from build123d import *

# Parameters (mm, degrees)
F0_W     = 580
F0_H     = 180
F1_DEPTH = 10
F2_W     = 560
F2_H     = 180
F2_W_2   = 540
F2_H_2   = 160
F3_DEPTH = 5


with BuildPart() as f1:
    # F0 (on Top) → F1 (new body)
    with BuildSketch(Plane.XY):
        Rectangle(F0_W, F0_H)
    extrude(amount=F1_DEPTH)

    # F2 (on face) → F3 (cut)
    with BuildSketch(Plane.XY.offset(10)):
        Rectangle(F2_W, F2_H)
        Rectangle(F2_W_2, F2_H_2, mode=Mode.SUBTRACT)
    extrude(amount=-F3_DEPTH, mode=Mode.SUBTRACT)


solid = f1.part
Can you work these out from the model? Positions are in its coordinate system, mm. Give positions to 0.01 mm unless a question says otherwise; leave off trailing zeros. Loops run counter-clockwise (first coordinate to the right, second up) from the corner with the lowest first, then second, coordinate; pieces in that order, holes last. Notation, with made-up numbers: (45.5, 57.25) -> (59.5, 57.25) arc R8 ccw to (59.5, 65.25) -> close; hole circle Ø9 at (15, 54.5). An arc over 180 degrees is marked (long way). Write item = value, one per line.
1) I need wall thicknesses on L1, parallel to X at y = 41, z = 8.75; L2, parallel to Z at x = -94, y = 81.5; L3, parallel to Y at x = -247.5, z = 6.5. Which ranges of each line are inside material? Lowest first, please. Write a range as from..to.
Check result:
L1 = -290..-280, -270..270, 280..290
L2 = 0..5
L3 = -80..80
2) Will these pins go through, and if not, where does the flat tip stop? pin 1 (5.5 mm diameter, centred on x = 25, z = 8, fed in from -Y); pin 2 (2.5 mm diameter, centred on x = -95.5, z = 8, fed in from +Y).
Check result:
pin_1 = -80
pin_2 = 80
3) Suppose I cut it at A-A on x = -28.5. Write out the boundary of the cut face in (y, z).
Check result:
outline = (-90, 0) -> (90, 0) -> (90, 5) -> (80, 5) -> (80, 10) -> (-80, 10) -> (-80, 5) -> (-90, 5) -> close
4) Thinking about a two-plate mould opening in X: for faces 1 (the flat face through (-290, -1, 5)), 2 (the flat face through (-84.3, 80.4, 5)), 3 (the flat face through (290, -1, 5)), 4 (the flat face through (-285, 1, 10)), which applies, released by +X, released by -X, zero draft, split by the parting line, or undercut?
Check result:
face_1 = released by -X
face_2 = undercut
face_3 = released by +X
face_4 = zero draft
5) Suppose I cut it at B-B on y = 40.5. Write out the boundary of the cut face in (x, z), then the cut area to 3 significant figures.
Check result:
outline = (-290, 0) -> (290, 0) -> (290, 10) -> (280, 10) -> (280, 5) -> (270, 5) -> (270, 10) -> (-270, 10) -> (-270, 5) -> (-280, 5) -> (-280, 10) -> (-290, 10) -> close
area = 5,700 mm2
